Source: CAD feature listing. Evaluate the final solid. Frame: model axes, mm. A direction names the side the tool comes from. Round coordinates to 2 decimals unless told otherwise and drop trailing zeros. Loops run counter-clockwise (first coordinate to the right, second up) from the corner with the lowest first, then second, coordinate; pieces in that order, holes last.
(1) Section A-A, the plane x = -26.5. Return the cut outline in (y, z), plus the area to 3 significant figures.
(2) Section C-C, the plane z = 2.5. Return the cut outline in (x, y), plus the area to 3 significant figures.
(3) Section B-B, the plane y = -0.05. Return the cut outline in (x, z), plus the area to 3 significant figures.
(4) Set-up query: faces 1 (the flat face through (0, 0.25, 0)), 2 (the flat face through (45, 0.5, 5)). Return all of +Z, -Z, +X, -X, +Y, -Y with unobstructed straight access to the full face (end or side cutting, diameter ignored); none if empty.
(5) Material intervals for probe 1 along Z at (x, y) = (25, -0.15); probe 2 along X at (y, z) = (-0.1, 3.75); probe 3 along X at (y, z) = (0.1, 5.25), sorted ascending.
(6) First-contact query: pin 1 Ø4 at (x, z) = (-8, 3) entering from +Y. Flat tip, straight axial feed; report the tip coordinate or a pass-through.
```python
from build123d import *

# Parameters (mm, degrees)
SKETCH2_W           = 1
SKETCH2_H           = 0.5
SKETCH3_W           = 3
SKETCH3_H           = 3
BOSS_EXTRUDE1_DEPTH = 0.75


with BuildPart() as part:
    # Sweep1: sweep along a path in Sketch1
    with BuildLine(Plane(origin=(0, 0, 0), x_dir=(1, 0, 0), z_dir=(0, 1, 0))) as sweep1_path:
        Line((-46.555555556, 5), (-40.555555556, 5))
        Line((-40.555555556, 5), (39.444444444, 5))
        Line((39.444444444, 5), (39.444444444, 0))
        Line((39.444444444, 0), (-40.555555556, 0))
        Line((-40.555555556, 0), (-40.555555556, -5))
        Line((-40.555555556, -5), (39.444444444, -5))
        Line((39.444444444, -5), (45.444444444, -5))
    # Sketch2 → Sweep1 (sweep)
    with BuildSketch(Plane(origin=(45.444444444, 0, 0), x_dir=(0, 0, -1), z_dir=(1, 0, 0))):
        with Locations((-5, 0)):
            Rectangle(SKETCH2_W, SKETCH2_H)
    sweep(path=sweep1_path.line, transition=Transition.RIGHT)

    # Sketch3 → Boss-Extrude1 (add)
    with BuildSketch(Plane.XZ.offset(0.25)):
        with Locations((-46.555555556, -5)):
            Rectangle(SKETCH3_W, SKETCH3_H)
        with Locations((45.444444444, 5)):
            Rectangle(SKETCH3_W, SKETCH3_H)
    extrude(amount=-BOSS_EXTRUDE1_DEPTH)


solid = part.part
```
Output values:
1. outline: (-0.25, -5.5) - (0.25, -5.5) - (0.25, -4.5) - (-0.25, -4.5) - close; (-0.25, -0.5) - (0.25, -0.5) - (0.25, 0.5) - (-0.25, 0.5) - close; (-0.25, 4.5) - (0.25, 4.5) - (0.25, 5.5) - (-0.25, 5.5) - close
1. area: 1.50 mm2
2. outline: (-41.06, -0.25) - (-40.06, -0.25) - (-40.06, 0.25) - (-41.06, 0.25) - close
2. area: 0.500 mm2
3. outline: (-48.06, -6.5) - (-45.06, -6.5) - (-45.06, -5.5) - (39.94, -5.5) - (39.94, 0.5) - (-40.06, 0.5) - (-40.06, 4.5) - (43.94, 4.5) - (43.94, 3.5) - (46.94, 3.5) - (46.94, 6.5) - (43.94, 6.5) - (43.94, 5.5) - (-41.06, 5.5) - (-41.06, -0.5) - (38.94, -0.5) - (38.94, -4.5) - (-45.06, -4.5) - (-45.06, -3.5) - (-48.06, -3.5) - close
3. area: 277 mm2
4. face 1: +Z, -Z, +Y
4. face 2: +Z, -Z, +X, -X, +Y
5. probe 1: z = -5.5 to -4.5, -0.5 to 0.5, 4.5 to 5.5
5. probe 2: x = -41.06 to -40.06, 43.94 to 46.94
5. probe 3: x = -41.06 to 46.94
6. pin 1: stops at y = 0.25
